Autodesk Inventor part; units mm, degrees
ref_plane "YZ Plane" through (0, 0, 0) normal (1, 0, 0) x (0, 1, 0)
ref_plane "XZ Plane" through (0, 0, 0) normal (0, 1, 0) x (-1, 0, 0)
ref_plane "XY Plane" through (0, 0, 0) normal (0, 0, 1) x (1, 0, 0)
sketch "Sketch1" plane through (0, 0, 0) normal (0, 0, 1) x (1, 0, 0)
  line L0 (-10, -15.65) -> (-10, 15.65)
  line L1 (-10, 15.65) -> (10, 15.65)
  line L2 (10, 15.65) -> (10, -15.65)
  line L3 (10, -15.65) -> (-10, -15.65)
  line L4 (1.5877, -12.1184) -> (1.5877, -10.9726)
  line L5 (5.119, -12.1184) -> (1.5877, -12.1184)
  line L6 (5.119, 11.1491) -> (5.119, -12.1184)
  line L7 (2.2936, 11.1491) -> (5.119, 11.1491)
  line L8 (2.2936, 12.739) -> (2.2936, 11.1491)
  line L9 (-2.2936, 12.739) -> (2.2936, 12.739)
  line L10 (-2.2936, 11.1491) -> (-2.2936, 12.739)
  line L11 (-5.119, 11.1491) -> (-2.2936, 11.1491)
  line L12 (-5.119, -12.1184) -> (-5.119, 11.1491)
  line L13 (-1.5877, -12.1184) -> (-5.119, -12.1184)
  line L14 (-1.5877, -10.9726) -> (-1.5877, -12.1184)
  line L15 (-4.1285, -10.9726) -> (-1.5877, -10.9726)
  line L16 (-4.1285, 10.0169) -> (-4.1285, -10.9726)
  line L17 (4.1285, 10.0169) -> (-4.1285, 10.0169)
  line L18 (4.1285, -10.9726) -> (4.1285, 10.0169)
  line L19 (1.5877, -10.9726) -> (4.1285, -10.9726)
  line L20 (2.9107, -1.4409) -> (2.9107, -4.3502)
  line L21 (-2.9107, -1.4409) -> (2.9107, -1.4409)
  line L22 (-2.9107, -4.3502) -> (-2.9107, -1.4409)
  line L23 (2.9107, -4.3502) -> (-2.9107, -4.3502)
  line L24 (2.9107, 7.9067) -> (2.9107, 4.9905)
  line L25 (-2.9107, 7.9067) -> (2.9107, 7.9067)
  line L26 (-2.9107, 4.9905) -> (-2.9107, 7.9067)
  line L27 (2.9107, 4.9905) -> (-2.9107, 4.9905)
  line L28 (2.9107, 3.2342) -> (2.9107, 0.4013)
  line L29 (-2.9107, 3.2342) -> (2.9107, 3.2342)
  line L30 (-2.9107, 0.4013) -> (-2.9107, 3.2342)
  line L31 (2.9107, 0.4013) -> (-2.9107, 0.4013)
  line L32 (2.9107, -6.1253) -> (2.9107, -8.9213)
  line L33 (-2.9107, -6.1253) -> (2.9107, -6.1253)
  line L34 (-2.9107, -8.9213) -> (-2.9107, -6.1253)
  line L35 (2.9107, -8.9213) -> (-2.9107, -8.9213)
  line L36 (-2.5, 20.75) -> (-8.5, 20.75)
  line L37 (-2.5, 21.75) -> (-2.5, 20.75)
  line L38 (2.5, 21.75) -> (-2.5, 21.75)
  line L39 (2.5, 20.75) -> (2.5, 21.75)
  line L40 (8.5, 20.75) -> (2.5, 20.75)
  line L41 (8.5, 15.65) -> (8.5, 20.75)
  line L42 (-8.5, 15.65) -> (8.5, 15.65)
  line L43 (-8.5, 20.75) -> (-8.5, 15.65)
  circle A0 centre (0, 18) radius 1.2
  line L44 (-8.5, -15.65) -> (-8.5, -20.75)
  line L45 (8.5, -15.65) -> (-8.5, -15.65)
  line L46 (8.5, -20.75) -> (8.5, -15.65)
  line L47 (2.5, -20.75) -> (8.5, -20.75)
  line L48 (2.5, -21.75) -> (2.5, -20.75)
  line L49 (-2.5, -21.75) -> (2.5, -21.75)
  line L50 (-2.5, -20.75) -> (-2.5, -21.75)
  line L51 (-8.5, -20.75) -> (-2.5, -20.75)
  circle A1 centre (0, -18) radius 1.2
  line L52 (12, 22.75) -> (-12, 22.75)
  line L53 (-12, 22.75) -> (-12, -22.75)
  line L54 (-12, -22.75) -> (12, -22.75)
  line L55 (12, -22.75) -> (12, 22.75)
  point P0 (0, 0)
  dimension "d0" = 2
  dimension "d1" = 2
  dimension "d2" = 2
  dimension "d3" = 2
extrude "Extrusion1" add sketch "Sketch1" against normal blind 8 contours L55 L54 L53 L52
ref_plane "Work Plane1" through (0, -22.75, 0) normal (-1, 0, 0) x (0, 0, 1)
sketch "Sketch2" plane through (0, -22.75, 0) normal (-1, 0, 0) x (0, 0, 1)
  line L0 (0, 44.5) -> (-8, 44.5)
  line L1 (-8, 0) -> (-8, 45.5)
  line L2 (-2, 44.5) -> (-8, 44.5)
  line L3 (-8, 44.5) -> (-8, 39)
  line L4 (-8, 39) -> (-2, 39)
  line L5 (-2, 39) -> (-2, 44.5)
  line L6 (-8, 38.4) -> (-8, 7.1)
  line L7 (-8, 22.75) -> (6.4462, 22.75)
  line L8 (0, 1) -> (-8, 1)
  line L9 (-2, 1) -> (-8, 1)
  line L10 (-8, 1) -> (-8, 6.5)
  line L11 (-8, 6.5) -> (-2, 6.5)
  line L12 (-2, 6.5) -> (-2, 1)
  point P0 (0, 22.75)
extrude "Extrusion2" add sketch "Sketch2" along normal mid plane 24
sketch "Sketch3" plane through (0, 0, -8) normal (0, 0, -1) x (-1, 0, 0)
  line L0 (-12, 22.75) -> (-12, -22.75)
  line L1 (-12, 22.75) -> (12, 22.75)
  line L2 (12, 22.75) -> (12, -22.75)
  line L3 (12, -22.75) -> (-12, -22.75)
  line L4 (-12, -22.75) -> (-12, 22.75)
  line L5 (-6, -13) -> (6, -13)
  line L6 (6, -13) -> (6, 13)
  line L7 (6, 13) -> (-6, 13)
  line L8 (-6, 13) -> (-6, -13)
  point P0 (0, 0)
extrude "Extrusion3" add sketch "Sketch3" along normal blind 2
chamfer "Chamfer1" distance 1 angle 45 4 edges at (0, 13, -10) (-6, 0, -10) (6, 0, -10) (0, -13, -10) measured on face at (-10, 4.3333, -10)
equation "\"d1\" = d0"
equation "\"d2\" = d1"
equation "\"d3\" = d1"
properties part number "battery indicator case"
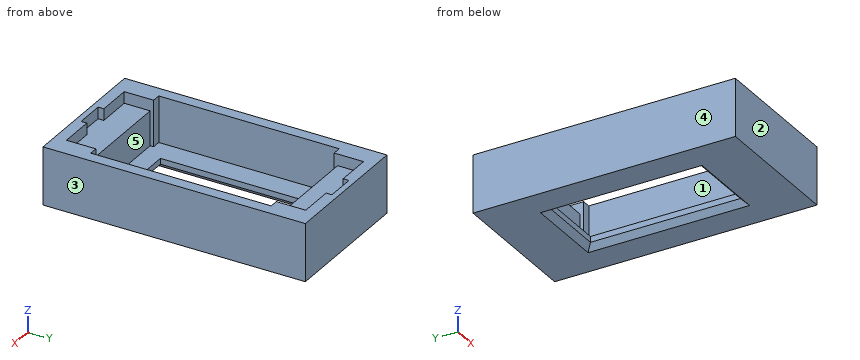
Geometry check sheet. Reference: the model listing, model coordinates, mm. Face numbers are marked on the shaded views. A direction names the side the tool comes from. Give positions to 0.01 mm unless a question says otherwise; leave off trailing zeros. Order: outer loops, then holes, each group sorted by start corner. A loop starts at its lowest first (then second) coordinate and runs counter-clockwise, first axis right, second up. Notation, with made-up numbers: (-10.75, 18.25) - (43.25, 18.25) arc R21 cw to (43.25, 33.25) - close; hole circle Ø5 at (38, 19.25). An arc over 180 degrees is marked (long way). Answer in a Markdown table with one row per item. Add a question column.
Q1. Cross-section at B-B, the plane x = -4.5. Enter the section's corners in (y, z), then the cut area to 3 significant figures.
Q2. Gauge pin test, flat end, axial feed: pin 1 (6 mm diameter, centred on x = 3.5, y = -18, fed in from +Z). Record the tip position at first contact, or that the pin passes through.
Q3. Mould release check, pull along X, two halves, no side actions. Record for the marked faces 1, 2 and 3: pulls with the +X half, pulls with the -X half, needs draft (parallel to the pull), parting line crosses it, or undercut.
Q4. Cross-section at D-D, the plane z = -1.25. Enter the section's corners in (x, y).
Q5. Tool access check on the marked faces 4 and 5. Record the directions out of +Z, -Z, +X, -X, +Y, -Y that give a thin tool (end or side, any length) a straight path to the whole face; none if there is none.
Q6. Material ranges on probe 1 along X at (y, z) = (-11.5, -1.5); probe 2 along Y at (x, z) = (1, -4); probe 3 along X at (y, z) = (16, -0.25), recorded low to high. Write a range as from..to.
Q7. Cross-section at C-C, the plane y = 2. Enter the section's corners in (x, z).
Q8. Cross-section at A-A, the plane z = -7.25. Enter the section's corners in (x, y), then the cut area to 3 significant figures.
Check values:
| question | item | result |
|---|---|---|
| 1 | outline | (-22.75, -10) - (-14, -10) - (-13, -9) - (-13, -8) - (-16.25, -8) - (-16.25, -2) - (-20.75, -2) - (-20.75, 0) - (-22.75, 0) - close; (13, -9) - (14, -10) - (22.75, -10) - (22.75, 0) - (20.75, 0) - (20.75, -2) - (16.25, -2) - (16.25, -8) - (13, -8) - close |
| 1 | area | 124 mm^2 |
| 2 | pin 1 | stops at z = 0 |
| 3 | face 1 | undercut |
| 3 | face 2 | needs draft |
| 3 | face 3 | pulls with the +X half |
| 4 | outline | (-12, -22.75) - (12, -22.75) - (12, 22.75) - (-12, 22.75) - close; hole (-10, -15.65) - (-8.5, -15.65) - (-8.5, -20.75) - (-2.5, -20.75) - (-2.5, -21.75) - (2.5, -21.75) - (2.5, -20.75) - (8.5, -20.75) - (8.5, -15.65) - (10, -15.65) - (10, 15.65) - (8.5, 15.65) - (8.5, 20.75) - (2.5, 20.75) - (2.5, 21.75) - (-2.5, 21.75) - (-2.5, 20.75) - (-8.5, 20.75) - (-8.5, 15.65) - (-10, 15.65) - close |
| 5 | face 4 | +Z, -Z, -X, +Y, -Y |
| 5 | face 5 | +Z |
| 6 | probe 1 | x = -12..-10, 10..12 |
| 6 | probe 2 | y = -22.75..-16.25, 16.25..22.75 |
| 6 | probe 3 | x = -12..-8.5, 8.5..12 |
| 7 | outline | (-12, -10) - (-7, -10) - (-6, -9) - (-6, -8) - (-10, -8) - (-10, 0) - (-12, 0) - close; (6, -9) - (7, -10) - (12, -10) - (12, 0) - (10, 0) - (10, -8) - (6, -8) - close |
| 8 | outline | (-12, -22.75) - (12, -22.75) - (12, 22.75) - (-12, 22.75) - close; hole (-10, -15.65) - (-8.5, -15.65) - (-8.5, -16.25) - (8.5, -16.25) - (8.5, -15.65) - (10, -15.65) - (10, 15.65) - (8.5, 15.65) - (8.5, 16.25) - (-8.5, 16.25) - (-8.5, 15.65) - (-10, 15.65) - close |
| 8 | area | 446 mm^2 |
